The model under review builds one solid part; all positions refer to its coordinate system, in mm. Face numbers are marked on the shaded views. A direction names the side the tool comes from. Give positions to 0.01 mm unless a question says otherwise; leave off trailing zeros. Loops run counter-clockwise (first coordinate to the right, second up) from the corner with the lowest first, then second, coordinate; pieces in that order, holes last. Notation, with made-up numbers: M 55.25,1.5 L 69.25,1.5 A18 ccw 69.25,5.5 Z; hole C 69,36.25 d1. An arc over 180 degrees is marked long. Put each result on its own line as item: value. Start each with the question number.
from build123d import *

# Parameters (mm, degrees)
SKETCH2_W                       = 27.178
SKETCH2_H                       = 21.59
INITIAL_EXTRUDE_DEPTH           = 6.35
SKETCH3_W                       = 27.178
SKETCH3_H                       = 1.27
INTIAL_EXTRUDE_HORIZONTAL_DEPTH = 12.192
SKETCH4_W                       = 27.178
SKETCH4_H                       = 1.27
SLIGHT_EXTRUDE_VERTICAL_DEPTH   = 0.254
SKETCH5_W                       = 3.048
SKETCH5_H                       = 21.59
CUT_EXTRUDE1_DEPTH              = 2.794
CUT_EXTRUDE2_REACH              = 33.537
SKETCH6_W                       = 1.379153921
SKETCH6_H                       = 12.954
SNAP_START                      = 11.473246079
SNAP_HOOK2_DEPTH                = 0.7366
SNAP_START_2                    = 8.31223189
SNAP_HOOK2_2_DEPTH              = 8.568362063
SNAP_START_3                    = 8.179116131
SNAP_HOOK2_3_DEPTH              = 8.834593581
SNAP_START_4                    = 9
SNAP_HOOK2_4_DEPTH              = 6
BOSS_EXTRUDE1_DEPTH             = 2.54
SKETCH8_W                       = 24.419692158
SKETCH8_H                       = 7.195933706
CUT_EXTRUDE3_DEPTH              = 0.762
SKETCH9_W                       = 24.419692158
SKETCH9_H                       = 20.32
BOSS_EXTRUDE2_DEPTH             = 2.794
SKETCH10_R                      = 5.08
CUT_EXTRUDE4_DEPTH              = 5.08


with BuildPart() as part:
    # Sketch2 → Initial Extrude (new body)
    with BuildSketch(Plane.XY):
        Rectangle(SKETCH2_W, SKETCH2_H)
    extrude(amount=INITIAL_EXTRUDE_DEPTH)

    # Sketch3 → Intial Extrude horizontal (add)
    with BuildSketch(Plane.XY.offset(6.35)):
        with Locations((0, 10.16)):
            Rectangle(SKETCH3_W, SKETCH3_H)
    extrude(amount=INTIAL_EXTRUDE_HORIZONTAL_DEPTH)

    # Sketch4 → Slight Extrude vertical (add)
    with BuildSketch(Plane.XZ.offset(-9.525)):
        with Locations((0, 17.907)):
            Rectangle(SKETCH4_W, SKETCH4_H)
    extrude(amount=SLIGHT_EXTRUDE_VERTICAL_DEPTH)

    # Sketch5 → Cut-Extrude1 (cut)
    with BuildSketch(Plane.ZY.offset(13.589)):
        with Locations((4.064, 0)):
            Rectangle(SKETCH5_W, SKETCH5_H)
    cut_extrude1 = extrude(amount=-CUT_EXTRUDE1_DEPTH, mode=Mode.SUBTRACT)

    # Mirror3: Cut-Extrude1 across plane
    add(cut_extrude1.mirror(Plane(origin=(0, 0, 0), x_dir=(0, 0, 1), z_dir=(1, 0, 0))), mode=Mode.SUBTRACT)

    # Sketch6 → Cut-Extrude2 (cut, up to next)
    with BuildSketch(Plane(origin=(0, 10.795, 0), x_dir=(1, 0, 0), z_dir=(0, 1, 0)), mode=Mode.PRIVATE) as cut_extrude2_sk1:
        with Locations((12.89942304, -12.065)):
            Rectangle(SKETCH6_W, SKETCH6_H)
    cut_extrude2_tool1 = extrude(cut_extrude2_sk1.sketch, amount=-CUT_EXTRUDE2_REACH, mode=Mode.PRIVATE) & part.part
    cut_extrude2 = cut_extrude2_tool1.solids().sort_by_distance((12.899423, 10.795, 12.065))[0]
    add(cut_extrude2, mode=Mode.SUBTRACT)

    # Mirror7: Cut-Extrude2 across plane
    add(cut_extrude2.mirror(Plane(origin=(0, 0, 0), x_dir=(0, 0, 1), z_dir=(1, 0, 0))), mode=Mode.SUBTRACT)

    # Snap Hook2: read off the stored shape, not the designer's step
    # Snap Hook2 outline → Snap Hook2 (add)
    with BuildSketch(Plane.YZ.offset(SNAP_START)):
        Polygon((10.795, 17.013709712), (10.795, 8.179116131), (15.113, 8.405412922), (15.113, 16.787412922), align=None)
    snap_hook2 = extrude(amount=SNAP_HOOK2_DEPTH)

    # Snap Hook2 2 outline → Snap Hook2 2 (add)
    with BuildSketch(Plane.XY.offset(SNAP_START_2)):
        Polygon((11.473246079, 10.795), (11.473246079, 15.113), (10.177846079, 10.795), align=None)
        Polygon((12.209846079, 15.113), (12.209846079, 13.335), (14.241846079, 13.335), (14.241846079, 14.605), align=None)
    snap_hook2_2 = extrude(amount=SNAP_HOOK2_2_DEPTH)

    # Snap Hook2 3 outline → Snap Hook2 3 (add)
    with BuildSketch(Plane.XY.offset(SNAP_START_3)):
        Polygon((11.473246079, 10.795), (11.473246079, 15.113), (10.177846079, 10.795), align=None)
    snap_hook2_3 = extrude(amount=SNAP_HOOK2_3_DEPTH)

    # Snap Hook2 4 outline → Snap Hook2 4 (cut)
    with BuildSketch(Plane.YZ.offset(SNAP_START_4)):
        Polygon((10.795, 8.179116131), (17, 8.179116131), (17, 8.504306402), (15.113, 8.405412922), align=None)
        Polygon((15.113, 16.787412922), (17, 16.688519443), (17, 17.013709712), (10.795, 17.013709712), align=None)
    snap_hook2_4 = extrude(amount=SNAP_HOOK2_4_DEPTH, mode=Mode.SUBTRACT)

    # Mirror6: Snap Hook2, Snap Hook2 2, Snap Hook2 3, Snap Hook2 4 across plane
    add(snap_hook2.mirror(Plane(origin=(0, 0, 0), x_dir=(0, 0, 1), z_dir=(1, 0, 0))))
    add(snap_hook2_2.mirror(Plane(origin=(0, 0, 0), x_dir=(0, 0, 1), z_dir=(1, 0, 0))))
    add(snap_hook2_3.mirror(Plane(origin=(0, 0, 0), x_dir=(0, 0, 1), z_dir=(1, 0, 0))))
    add(snap_hook2_4.mirror(Plane(origin=(0, 0, 0), x_dir=(0, 0, 1), z_dir=(1, 0, 0))), mode=Mode.SUBTRACT)

    # Sketch7 → Boss-Extrude1 (add)
    with BuildSketch(Plane(origin=(0, 10.795, 0), x_dir=(1, 0, 0), z_dir=(0, 1, 0))):
        Polygon((-8.962447439, -8.179116131), (-8.962447439, -18.542), (8.962447439, -18.542), (8.962447439, -8.179116131), (9, -8.179116131), (10.177846079, -8.179116131), (12.209846079, -8.179116131), (12.209846079, -5.588), (10.795, -5.588), (10.795, -2.54), (13.589, -2.54), (13.589, 0), (-13.589, 0), (-13.589, -2.54), (-10.795, -2.54), (-10.795, -5.588), (-12.209846079, -5.588), (-12.209846079, -8.179116131), (-10.177846079, -8.179116131), (-9, -8.179116131), align=None)
    extrude(amount=BOSS_EXTRUDE1_DEPTH)

    # Sketch8 → Cut-Extrude3 (cut)
    with BuildSketch(Plane.XZ.offset(-9.525)):
        with Locations((0, 13.674033147)):
            Rectangle(SKETCH8_W, SKETCH8_H)
    extrude(amount=-CUT_EXTRUDE3_DEPTH, mode=Mode.SUBTRACT)

    # Sketch9 → Boss-Extrude2 (add)
    with BuildSketch(Plane.XY.offset(6.35)):
        with Locations((0, -0.635)):
            Rectangle(SKETCH9_W, SKETCH9_H)
    extrude(amount=BOSS_EXTRUDE2_DEPTH)

    # Sketch10 → Cut-Extrude4 (cut)
    with BuildSketch(Plane(origin=(0, 13.335, 0), x_dir=(1, 0, 0), z_dir=(0, 1, 0))):
        with Locations(Location((0, -12.7, 0), (0, 0, 270))):
            Circle(SKETCH10_R)
    extrude(amount=-CUT_EXTRUDE4_DEPTH, mode=Mode.SUBTRACT)


solid = part.part
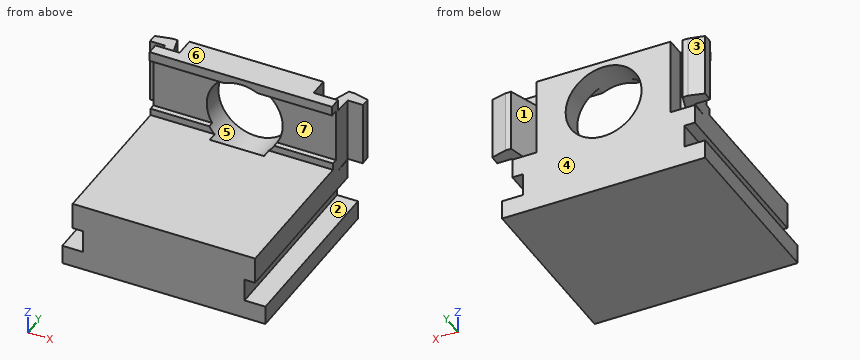
(1) For the marked faces 5, 6 and 7, list the 3-axis set-ups (+Z, -Z, +X, -X, +Y, -Y) from which the entire face can be reached by the end or side of a thin tool; tool diameter is ignored.
(2) We need section B-B, the plane x = 0. Write out the cut boundary in (y, z) (3 decimals), plus the area to 3 significant figures.
(3) To check wall thickness, follow L1, parallel to X at y = 10.65, z = 12.7; L2, parallel to X at y = 11.4, z = 12.7; L3, parallel to Y at x = -3, z = 17.5 (3 decimals). State the ranges of each line that lie inside material, in increasing order. Write a range as [from, to].
(4) Draft analysis for pull direction X (two halves, no side actions). For the marked faces 1, 2, 3 and 4, state which applies: +X half, -X half, draft (parallel to the pull), parting line (faces both ways), or undercut.
(5) Insertion check: pin 1 (3.5 mm diameter, centred on x = 9, z = 13, fed in from -Y); pin 2 (8 mm diameter, centred on x = -8.5, z = 15, fed in from -Y); pin 3 (0.8 mm diameter, centred on y = 12.5, z = 11.5, fed in from +X). Each pin has a flat end and moves straight along its axis. Give the tip position at first contact, or say it passes through.
(6) We need section C-C, the plane x = 9.75. Write out the cut boundary in (y, z) (3 decimals), plus the area to 3 significant figures.
(7) We need section D-D, the plane y = -2. Write out the cut boundary in (x, z) (3 decimals), plus the area to 3 significant figures.
(8) We need section A-A, the plane z = 12.7. Write out the cut boundary in (x, y) (3 decimals).
Check sheet entries:
1. face 5: +Y
1. face 6: +Z, +X, -X, +Y, -Y
1. face 7: +X, -X, -Y
2. outline: M -10.795,0 L 13.335,0 L 13.335,7.62 L 8.255,7.62 L 8.255,9.144 L -10.795,9.144 Z; M 9.271,17.78 L 13.335,17.78 L 13.335,18.542 L 9.271,18.542 Z
2. area: 216 mm²
3. L1: x = [-12.21, -5.08], [5.08, 12.21]
3. L2: x = [-12.21, -10.36], [-8.96, -5.08], [5.08, 8.96], [10.36, 12.21]
3. L3: y = [9.271, 13.335]
4. face 1: undercut
4. face 2: draft
4. face 3: -X half
4. face 4: undercut
5. pin 1: stops at y = 10.29
5. pin 2: stops at y = 9.27
5. pin 3: stops at x = 12.21
6. outline: M -10.795,0 L 13.335,0 L 13.335,8.179 L 10.795,8.179 L 10.795,18.542 L 9.271,18.542 L 9.271,17.272 L 10.287,17.272 L 10.287,10.076 L 9.525,10.076 L 9.525,9.144 L -10.795,9.144 Z
6. area: 225 mm²
7. outline: M -13.589,0 L 13.589,0 L 13.589,2.54 L 10.795,2.54 L 10.795,5.588 L 12.21,5.588 L 12.21,9.144 L -12.21,9.144 L -12.21,5.588 L -10.795,5.588 L -10.795,2.54 L -13.589,2.54 Z
7. area: 222 mm²
8. outline: M -14.242,13.335 L -12.21,13.335 L -12.21,10.287 L -5.08,10.287 L -5.08,13.335 L -8.962,13.335 L -8.962,10.795 L -10.178,10.795 L -11.473,15.113 L -12.21,15.113 L -14.242,14.605 Z; M 5.08,10.287 L 12.21,10.287 L 12.21,13.335 L 14.242,13.335 L 14.242,14.605 L 12.21,15.113 L 11.473,15.113 L 10.178,10.795 L 8.962,10.795 L 8.962,13.335 L 5.08,13.335 Z
